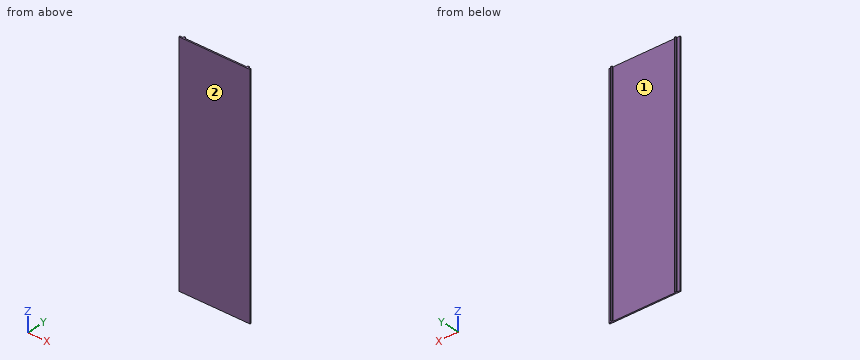
```python
from build123d import *

# Parameters (mm, degrees)
SKETCH_1_W      = 104
SKETCH_1_H      = 340
EXTRUDE_1_DEPTH = 2
SKETCH_2_W      = 2
SKETCH_2_H      = 2
EXTRUDE_2_DEPTH = 340


with BuildPart() as part:
    # Эскиз1 → Бобышка-Вытянуть1 (new body)
    with BuildSketch(Plane(origin=(0, 0, 0), x_dir=(1, 0, 0), z_dir=(0, 1, 0))):
        Rectangle(SKETCH_1_W, SKETCH_1_H)
    extrude(amount=EXTRUDE_1_DEPTH)

    # Эскиз2 → Бобышка-Вытянуть2 (add)
    with BuildSketch(Plane.XY.offset(170)):
        with Locations((-46.7, 3)):
            Rectangle(SKETCH_2_W, SKETCH_2_H)
    extrude_2 = extrude(amount=-EXTRUDE_2_DEPTH)

    # Зеркальное отражение1: Бобышка-Вытянуть2 across plane
    add(extrude_2.mirror(Plane(origin=(0, 0, 0), x_dir=(0, 0, 1), z_dir=(1, 0, 0))))


solid = part.part
```
Check sheet for the modelled part. Datum: model origin and axes. Units: mm. Face numbers are marked on the shaded views. Coordinates: 2 decimals unless noted, no trailing zeros. Loops run counter-clockwise (first coordinate to the right, second up) from the corner with the lowest first, then second, coordinate; pieces in that order, holes last.
1) Sectioned sample at C-C (x = -41.5). Record the boundary of the cut face in (y, z).
2) Material ranges on probe 1 along X at (y, z) = (3.6, -8.5); probe 2 along Y at (x, z) = (22, -58), recorded low to high.
3) Sectioned sample at B-B (z = -20). Record the boundary of the cut face in (x, y), and give its area (3 significant figures).
4) Release check for a two-part mould opening along X. For the marked faces 1 and 2 record: released by +X, released by -X, zero draft, split by the parting line, or undercut.
5) Gauge pin test, flat ends, axial feed: pin 1 (4.5 mm diameter, centred on x = 50, z = 58.5, fed in from +Y); pin 2 (0.6 mm diameter, centred on y = 3, z = -59, fed in from +X). Record the tip position at first contact, or that the pin passes through.
6) Sectioned sample at A-A (y = 2.85). Record the boundary of the cut face in (x, z), and give its area (3 significant figures).
Check sheet entries:
1. outline: (0, -170) - (2, -170) - (2, 170) - (0, 170) - close
2. probe 1: x = -47.7 to -45.7, 45.7 to 47.7
2. probe 2: y = 0 to 2
3. outline: (-52, 0) - (52, 0) - (52, 2) - (47.7, 2) - (47.7, 4) - (45.7, 4) - (45.7, 2) - (-45.7, 2) - (-45.7, 4) - (-47.7, 4) - (-47.7, 2) - (-52, 2) - close
3. area: 216 mm2
4. face 1: undercut
4. face 2: zero draft
5. pin 1: stops at y = 2
5. pin 2: stops at x = 47.7
6. outline: (-47.7, -170) - (-45.7, -170) - (-45.7, 170) - (-47.7, 170) - close; (45.7, -170) - (47.7, -170) - (47.7, 170) - (45.7, 170) - close
6. area: 1,360 mm2
